Source: CAD feature listing. Evaluate the final solid. Frame: model axes, mm. A direction names the side the tool comes from. Coordinates: 2 decimals unless noted, no trailing zeros. Write each loop counter-clockwise with the first axis right and the second up, starting at its lowest first coordinate (ties: lowest second). Pieces come first, ordered by that corner, then holes. Notation, with made-up numbers: M 3,-28 L 49,-28 A17 ccw 49,3 Z; hole C -23.5,71 d2. An arc over 180 degrees is marked long. Answer as CSV lines item,"result". Start each with the question number.
1. Line query: probe 1 along Y at (x, z) = (164, 16); probe 2 along Y at (x, z) = (6, 22); probe 3 along X at (y, z) = (138, 28). Output: solid intervals per line, ascending. Write a range as [from, to].
2. Section A-A on x = 145. Return the cut outline in (y, z), plus the area to 3 significant figures.
3. Contact query for flat-ended pins moving along their axis: pin 1 Ø4.5 at (x, z) = (162.5, 13.5) entering from +Y; pin 2 Ø4.5 at (x, y) = (164, 138) entering from +Z; pin 3 Ø8 at (x, z) = (124.5, 76) entering from -Y. Output: stop coordinate, or through.
4. Section C-C on z = 62. Return the cut outline in (x, y).
5. Reachability of faces 1 (the face through (140, 203, 185)), 2 (the face through (63, 170, 20)), 3 (the face through (84, 0, 20)), 4 (the face through (84, 99, 40)), 5 (the face through (163, 170, 20)) from +Z, -Z, +X, -X, +Y, -Y: full face, straight path, thin tool, end or side. Return the list, or none.
6. Section B-B on y = 191. Return the cut outline in (x, z), plus the area to 3 significant figures.
Autodesk Inventor part; units mm, degrees
ref_plane "YZ Plane" through (0, 0, 0) normal (1, 0, 0) x (0, 1, 0)
ref_plane "XZ Plane" through (0, 0, 0) normal (0, 1, 0) x (-1, 0, 0)
ref_plane "XY Plane" through (0, 0, 0) normal (0, 0, 1) x (1, 0, 0)
sketch "Sketch1" plane through (0, 0, 0) normal (0, 0, 1) x (1, 0, 0)
  line L0 (0, 0) -> (170, 0)
  line L1 (170, 0) -> (170, 170)
  line L2 (170, 170) -> (0, 170)
  line L3 (0, 170) -> (0, 0)
  circle A0 centre (6, 5) radius 2
  circle A1 centre (164, 5) radius 2
  circle A2 centre (164, 138) radius 2
  circle A3 centre (6, 160) radius 2
  line L4 (6, 5) -> (164, 5) construction
  point P0 (85, 5)
  point P1 (85, 0)
  dimension "d0" = 170
  dimension "d1" = 170
  dimension "d2" = 4
  dimension "d3" = 4
  dimension "d4" = 4
  dimension "d5" = 4
  dimension "d6" = 158
  dimension "d7" = 155
  dimension "d8" = 133
  dimension "d9" = 32
extrude "Extrusion1" add sketch "Sketch1" along normal blind 40
sketch "Sketch2" plane through (0, 0, 40) normal (0, 0, 1) x (1, 0, 0)
  line L0 (170, 170) -> (0, 170)
  line L1 (125, 170) -> (155, 170)
  line L2 (155, 170) -> (155, 210)
  line L3 (155, 210) -> (125, 210)
  line L4 (125, 210) -> (125, 170)
  line L5 (170, 0) -> (170, 170)
  point P0 (0, 0)
  dimension "d12" = 30
  dimension "d13" = 40
  dimension "d14" = 15
extrude "Extrusion2" add sketch "Sketch2" against normal blind 40 and the other way blind 145
sketch "Sketch3" plane through (155, 170, 0) normal (1, 0, 0) x (0, 0, -1)
  line L0 (-185, 0) -> (-40, 0)
  line L1 (-185, 0) -> (-40, 0)
  line L2 (-40, 0) -> (-40, 25)
  line L3 (-40, 25) -> (-185, 25)
  line L4 (-185, 25) -> (-185, 0)
  point P0 (0, -170)
  dimension "d19" = 25
extrude "Extrusion3" cut sketch "Sketch3" against normal through all
properties part number "NVIDIA Jetson TX2" material "ABS Plastic"
Values:
1,probe 1,"[0, 3], [7, 136], [140, 170]"
1,probe 2,"[0, 3], [7, 158], [162, 170]"
1,probe 3,"[0, 162], [166, 170]"
2,outline,"M 0,0 L 210,0 L 210,185 L 195,185 L 195,40 L 0,40 Z"
2,area,"10,600 mm²"
3,pin 1,"y = 170"
3,pin 2,"z = 40"
3,pin 3,"y = 195"
4,outline,"M 125,195 L 155,195 L 155,210 L 125,210 Z"
5,face 1,"+Z, +X, -X, +Y, -Y"
5,face 2,"+Z, -Z, -X, +Y"
5,face 3,"+Z, -Z, +X, -X, -Y"
5,face 4,"+Z, +X, -X, -Y"
5,face 5,"+Z, -Z, +X, +Y"
6,outline,"M 125,0 L 155,0 L 155,40 L 125,40 Z"
6,area,"1,200 mm²"
